The listing builds one solid part. Answer for the finished solid, in the listing's coordinates (mm). Face numbers are marked on the shaded views. Round coordinates to 2 decimals unless told otherwise and drop trailing zeros. Order: outer loops, then holes, each group sorted by start corner. A loop starts at its lowest first (then second) coordinate and runs counter-clockwise, first axis right, second up. Notation, with made-up numbers: (80, 47) -> (107, 47) arc R8 cw to (107, 52) -> close; hole circle Ø5 at (10, 84.5). An arc over 180 degrees is marked (long way). Return JSON: item names as keys, results as strings. Group by question number.
(1) Each of these flat-tipped pins is pushed along its axis until it touches: pin 1 (8 mm diameter, centred on x = 6.5, y = -30.5, fed in from +Z); pin 2 (9.5 mm diameter, centred on x = 1.5, z = 7.5, fed in from -Y); pin 3 (10 mm diameter, centred on y = 33.5, z = 15.5, fed in from +X). Where does it stop, or does it pass through?
(2) Determine the mould class of the marked faces 1, 2 and 3 for opening direction X: +X half, -X half, draft (parallel to the pull), parting line (faces both ways), or undercut.
(3) Consider line 1 (Z direction, x = 1, y = 39.5); line 2 (Y direction, x = -4, z = 79.5); line 3 (Y direction, x = 5.5, z = 72.5). Determine where each line is inside the solid, lowest interval first. Write a range as [from, to].
(4) The part is cut by section A-A (z = 101). Determine the outline of the cut face in (x, y), plus the area to 3 significant figures.
from build123d import *

# Parameters (mm, degrees)
F2_W            = 17
F2_H            = 4
F3_DEPTH        = 12
F3_COPIES_COUNT = 6
F4_R            = 0.59
F5_R            = 1.3


# Not quite as in the source:
# - a pattern or mirror of a feature is missing from the dataset's text; its kind, count and spacing are read off the source's solid


with BuildPart() as f1:
    # F0 (on Front) → F1 (revolve)
    with BuildSketch(Plane.XZ):
        Polygon((0, 110), (0, 40), (9, 0), (48, 0), (48, 13), (8, 13), (8, 110), align=None)
    revolve(axis=Axis((0, 0, 75), (0, 0, 1)))

    # F2 (on face) → F3 (cut)
    with BuildSketch(Plane(origin=(0, 0, 0), x_dir=(1, 0, 0), z_dir=(0, 0, -1))):
        with Locations((0, 43)):
            Rectangle(F2_W, F2_H)
    f3 = extrude(amount=-F3_DEPTH, mode=Mode.SUBTRACT)

    # F3_copies: F3 ×6 about axis
    f3_copies_axis = Axis((0, 0, 0), (0, 0, 1))
    for i in range(1, F3_COPIES_COUNT):
        add(f3.rotate(f3_copies_axis, i * 360 / F3_COPIES_COUNT), mode=Mode.SUBTRACT)

    # F4
    f4_edges = [f1.edges().sort_by_distance(p)[0] for p in [
        (-48, 0, 13),
    ]]
    fillet(f4_edges, radius=F4_R)

    # F5
    f5_edges = [f1.edges().sort_by_distance(p)[0] for p in [
        (-8, 0, 110),
    ]]
    fillet(f5_edges, radius=F5_R)


solid = f1.part
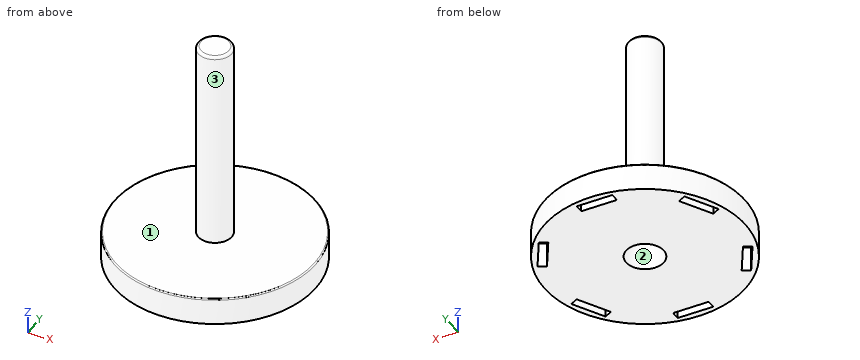
Answer below:
{
 "1": {"pin 1": "stops at z = 13", "pin 2": "stops at y = -48", "pin 3": "stops at x = 37.88"},
 "2": {"face 1": "draft", "face 2": "undercut", "face 3": "parting line"},
 "3": {"line 1": "z = [0, 13]", "line 2": "y = [-6.93, 6.93]", "line 3": "y = [-5.81, 5.81]"},
 "4": {"outline": "circle Ø16 at (0, 0)", "area": "201 mm²"}
}
